Autodesk Inventor part; units mm, degrees
ref_plane "YZ Plane" through (0, 0, 0) normal (1, 0, 0) x (0, 1, 0)
ref_plane "XZ Plane" through (0, 0, 0) normal (0, 1, 0) x (-1, 0, 0)
ref_plane "XY Plane" through (0, 0, 0) normal (0, 0, 1) x (1, 0, 0)
sketch "Skizze1" plane through (0, 0, 0) normal (0, 1, 0) x (-1, 0, 0)
  line L0 (-12.5, 19.9585) -> (-35, -16.0415)
  line L1 (-35, -16.0415) -> (-35, -81.0415)
  line L2 (-35, -81.0415) -> (-25, -81.0415)
  line L3 (-25, -81.0415) -> (-25, -26.0415)
  line L4 (-25, -26.0415) -> (-15, -10.0415)
  line L5 (-15, -10.0415) -> (15, -10.0415)
  line L6 (15, -10.0415) -> (25, -26.0415)
  line L7 (25, -26.0415) -> (25, -81.0415)
  line L8 (25, -81.0415) -> (35, -81.0415)
  line L9 (35, -81.0415) -> (35, -16.0415)
  line L10 (35, -16.0415) -> (12.5, 19.9585)
  line L11 (0, -101.2415) -> (0, 40.1585)
  line L12 (12.5, 19.9585) -> (-12.5, 19.9585)
  point P0 (0, 0)
  dimension "d0" = 10
  dimension "d1" = 10
  dimension "d4" = 30
  dimension "d5" = 15
  dimension "d6" = 70
  dimension "d7" = 55
  dimension "d8" = 55
  dimension "d9" = 65
  dimension "d10" = 65
  dimension "d11" = 10
  dimension "d13" = 25
  dimension "d14" = 30
  dimension "d15" = 30
  dimension "d16" = 50
extrude "Extrusion1" add sketch "Skizze1" along normal blind 25
sketch "Skizze2" plane through (-12.5, 0, 19.9585) normal (0, 0, 1) x (1, 0, 0)
  line L0 (-22.5, 25) -> (0, 25)
  line L1 (0, 0) -> (25, 0)
  line L2 (0, 25) -> (25, 25)
  line L3 (25, 25) -> (25, 0)
  line L4 (25, 0) -> (0, 0)
  line L5 (0, 0) -> (0, 25)
  point P0 (12.5, 0)
extrude "Extrusion2" add sketch "Skizze2" along normal blind 150
sketch "Skizze3" plane through (35, 0, -16.0415) normal (1, 0, 0) x (0, 0, -1)
  circle A0 centre (55, 12.5) radius 5.5
  circle A1 centre (25, 12.5) radius 5.5
  line L0 (-236.2, 0) -> (115.2, 0)
  line L1 (65, 0) -> (65, 25)
  point P0 (-16.0415, 0)
  dimension "d21" = 12.5
  dimension "d22" = 12.5
  dimension "d23" = 30
  dimension "d24" = 11
  dimension "d25" = 11
  dimension "d26" = 10
extrude "Extrusion3" cut sketch "Skizze3" against normal blind 300
fillet "Rundung1" radius 2 30 edges at (-20, 25, -18.0415) (0, 25, -10.0415) (-25, 25, -53.5415) (20, 25, -18.0415) (25, 25, -53.5415) (30, 25, -81.0415) (-30, 25, -81.0415) (-35, 25, -48.5415) (-23.75, 25, 1.9585) (23.75, 25, 1.9585) (12.5, 25, 94.9585) (-12.5, 25, 94.9585) (-25, 12.5, -81.0415) (-35, 12.5, -81.0415) (25, 12.5, -81.0415) (35, 12.5, -81.0415) (35, 25, -48.5415) (30, 0, -81.0415) (35, 0, -48.5415) (25, 0, -53.5415) (20, 0, -18.0415) (0, 0, -10.0415) (-20, 0, -18.0415) (-25, 0, -53.5415) (-30, 0, -81.0415) (-35, 0, -48.5415) (23.75, 0, 1.9585) (-23.75, 0, 1.9585) (-12.5, 0, 94.9585) (12.5, 0, 94.9585)
sketch "Skizze4" plane through (12.5, 2, 169.9585) normal (1, 0, 0) x (0, 0, -1)
  circle A0 centre (20, 10) radius 5
  circle A1 centre (100, 10) radius 5
  line L0 (0, 0) -> (0, 21)
  line L1 (0, -2) -> (150.5736, -2)
  point P0 (169.9585, -2)
  dimension "d31" = 10
  dimension "d32" = 10
  dimension "d33" = 20
  dimension "d34" = 80
  dimension "d35" = 12
  dimension "d36" = 12
extrude "Extrusion4" cut sketch "Skizze4" against normal blind 29
sketch "Skizze5" plane through (0, 0, 0) normal (0, -1, 0) x (1, 0, 0)
  circle A0 centre (0, 44.9585) radius 2.25
  circle A1 centre (0, 94.9585) radius 2.25
  line L0 (12.5, 19.9585) -> (12.5, 169.9585)
  line L1 (-10.5, 169.9585) -> (10.5, 169.9585)
  point P0 (0, 0)
  dimension "d39" = 4.5
  dimension "d40" = 4.5
  dimension "d41" = 50
  dimension "d42" = 12.5
  dimension "d43" = 12.5
  dimension "d44" = 75
extrude "Extrusion5" cut sketch "Skizze5" against normal blind 30
sketch "Skizze6" plane through (12.5, 2, 169.9585) normal (1, 0, 0) x (0, 0, -1)
  circle A0 centre (100, 10) radius 5
  circle A1 centre (100, 10) radius 7.4925
  circle A2 centre (20, 10) radius 5
  circle A3 centre (20, 10) radius 7.4925
  point P0 (169.9585, -2)
  dimension "d47" = 14.985
  dimension "d48" = 14.985
extrude "Extrusion6" cut sketch "Skizze6" against normal blind 5
sketch "Skizze7" plane through (-12.5, 2, 19.9585) normal (-1, 0, 0) x (0, 0, 1)
  circle A0 centre (130, 10) radius 5
  circle A1 centre (130, 10) radius 7.4925
  circle A2 centre (50, 10) radius 5
  circle A3 centre (50, 10) radius 7.4925
  point P0 (-19.9585, -2)
  dimension "d51" = 14.985
  dimension "d52" = 14.985
extrude "Extrusion7" cut sketch "Skizze7" against normal blind 5
properties part number "basisachse"
CAD build for the part. Positions are in the model's coordinates, mm. A direction names the side the tool comes from. Coordinates: 2 decimals unless noted, no trailing zeros. Order: outer loops, then holes, each group sorted by start corner. A loop starts at its lowest first (then second) coordinate and runs counter-clockwise, first axis right, second up.
(1) Saw through at D-D, the plane y = 9.5. Count the separate pieces of the cut face and the enclosed holes in it, and give its area (3 significant figures).
Solution:
separate pieces: 7
enclosed holes: 2
area: 5,670 mm2
(2) Saw through at B-B, the plane z = -59. Write the cut outline in (x, y), and give its area (3 significant figures).
Solution:
outline: (-35, 2) arc R2 ccw to (-33, 0) - (-27, 0) arc R2 ccw to (-25, 2) - (-25, 23) arc R2 ccw to (-27, 25) - (-33, 25) arc R2 ccw to (-35, 23) - close; (25, 2) arc R2 ccw to (27, 0) - (33, 0) arc R2 ccw to (35, 2) - (35, 23) arc R2 ccw to (33, 25) - (27, 25) arc R2 ccw to (25, 23) - close
area: 493 mm2
(3) Which spindle directions (+Z, -Z, +X, -X, +Y, -Y) get a long thin tool onto all of the face, cutting with end or side? Do faces 1 (the face through (20.27, 0.6, -17.39)), 2 (the face through (-10.035, 17.064, 64.436)), 3 (the face through (20.29, 24.43, -17.37)), 4 (the face through (0, 12, -10.042)). Say none if no direction does.
Solution:
face 1: -Z, -Y
face 2: -X
face 3: -Z, +Y
face 4: -Z, +Y, -Y
(4) Saw through at C-C, the plane z = 83. Write the cut outline in (x, y).
Solution:
outline: (-12.5, 2) arc R2 ccw to (-10.5, 0) - (10.5, 0) arc R2 ccw to (12.5, 2) - (12.5, 23) arc R2 ccw to (10.5, 25) - (-10.5, 25) arc R2 ccw to (-12.5, 23) - close
(5) Drill centre lines: L1, parallel to Z at x = 0, y = 16.5; L2, parallel to X at y = 16, z = -65.5; L3, parallel to Z at x = 10, y = 5.5. Where is each one in solid material? Low to high.
Solution:
L1: z = -10.04 to 42.71, 47.21 to 67.78, 72.14 to 92.71, 97.21 to 147.78, 152.14 to 169.96
L2: x = -35 to -25, 25 to 35
L3: z = -10.04 to 66.23, 73.69 to 146.23, 153.69 to 169.96
(6) Saw through at A-A, the plane x = 0. Write the cut outline in (y, z), and give its area (3 significant figures).
Solution:
outline: (0, -8.04) arc R2 ccw to (2, -10.04) - (23, -10.04) arc R2 ccw to (25, -8.04) - (25, 42.71) - (0, 42.71) - close; (0, 47.21) - (25, 47.21) - (25, 92.71) - (0, 92.71) - close; (0, 97.21) - (25, 97.21) - (25, 169.96) - (0, 169.96) - close; hole circle Ø10 at (12, 69.96); hole circle Ø10 at (12, 149.96)
area: 4,120 mm2
(7) Pin check, flat tips, straight feed: pin 1 Ø13.5 at (y, z) = (12, 149.96) entering from -X; pin 2 Ø1 at (y, z) = (18, 6) entering from -X; pin 3 Ø6 at (y, z) = (17.5, 115.5) entering from -X. Stop position of each tip, or through.
Solution:
pin 1: stops at x = -7.5
pin 2: stops at x = -21.54
pin 3: stops at x = -12.5
(8) Mould opens along Y. For faces 5 (the face through (7.5, 7, 148)), 6 (the face through (-3, 0, 54)), 7 (the face through (-30, 12, -81.042)) say: released by +Y, released by -Y, zero draft, split by the parting line, or undercut.
Solution:
face 5: undercut
face 6: released by -Y
face 7: zero draft
